Could you check a few things on this drawing? It's one solid part, dimensions in mm from its lowest x, y, z. Round coordinates to 2 decimals unless told otherwise and drop trailing zeros. Order: outer loops, then holes, each group sorted by start corner. A loop starts at its lowest first (then second) coordinate and runs counter-clockwise, first axis right, second up. Notation, with made-up numbers: (-26, -23.5) -> (-7, -23.5) arc R35 ccw to (-7, 8.5) -> close; hole circle Ø11 at (47, 42). An arc over 180 degrees is marked (long way). Use a Markdown table: item, result. Add a question column.
(1) I want a section at B-B, the plane x = 82.55. Please give me the cut outline in (y, z), then the cut area to 3 significant figures.
(2) If I drill on probe 1 along Y at (x, z) = (164.5, 241); probe 2 along Z at (x, y) = (89.5, 28); probe 3 along X at (y, z) = (25.5, 396), over which ranges is the centre line in solid material (lowest first)?
(3) I want a section at C-C, the plane x = 169.5. Please give me the cut outline in (y, z).
(4) Thinking about a two-plate mould opening in Z: for the marked faces 1 and 2, which applies, pulls with the +Z half, pulls with the -Z half, needs draft (parallel to the pull), parting line crosses it, or undercut?
(5) I want a section at A-A, the plane z = 381. Please give me the cut outline in (x, y), then the cut area to 3 significant figures.
(6) I'm going to push flat-ended pins straight in: P1, Ø5, axis at x = 57, y = 31, coming from the +Z side; P2, Ø5, axis at x = 121, z = 71.5, coming from the +Y side. Where does each tip first touch, or does it pass through?
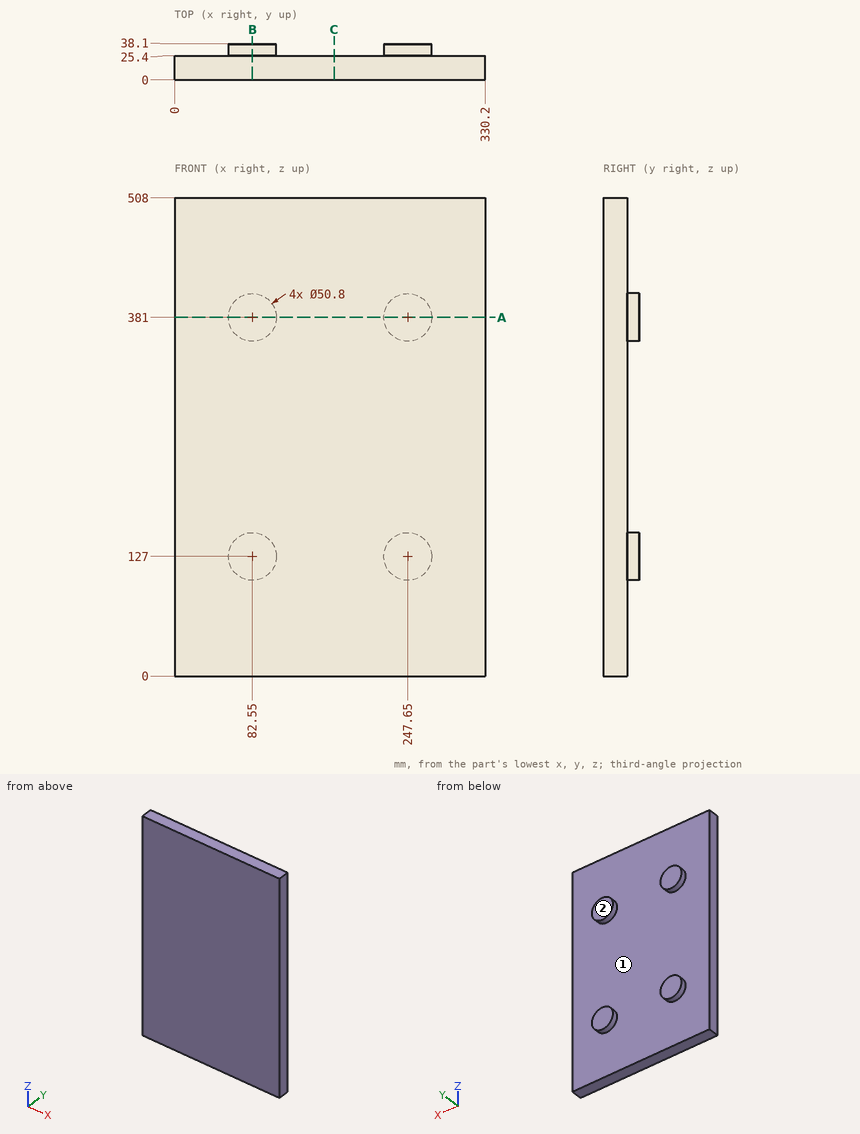
Taken from the geometry:
| question | item | result |
|---|---|---|
| 1 | outline | (0, 0) -> (25.4, 0) -> (25.4, 101.6) -> (38.1, 101.6) -> (38.1, 152.4) -> (25.4, 152.4) -> (25.4, 355.6) -> (38.1, 355.6) -> (38.1, 406.4) -> (25.4, 406.4) -> (25.4, 508) -> (0, 508) -> close |
| 1 | area | 14,200 mm2 |
| 2 | probe 1 | y = 0 to 25.4 |
| 2 | probe 2 | z = 102.57 to 151.43, 356.57 to 405.43 |
| 2 | probe 3 | x = 62.05 to 103.05, 227.15 to 268.15 |
| 3 | outline | (0, 0) -> (25.4, 0) -> (25.4, 508) -> (0, 508) -> close |
| 4 | face 1 | undercut |
| 4 | face 2 | needs draft |
| 5 | outline | (0, 0) -> (330.2, 0) -> (330.2, 25.4) -> (273.05, 25.4) -> (273.05, 38.1) -> (222.25, 38.1) -> (222.25, 25.4) -> (107.95, 25.4) -> (107.95, 38.1) -> (57.15, 38.1) -> (57.15, 25.4) -> (0, 25.4) -> close |
| 5 | area | 9,680 mm2 |
| 6 | P1 | stops at z = 391.67 |
| 6 | P2 | stops at y = 25.4 |
